Could you check a few things on this model? Use its own coordinates, in mm. Give positions to 0.01 mm unless a question says otherwise; leave off trailing zeros. Write each loop counter-clockwise with the first axis right and the second up, starting at its lowest first coordinate (ties: lowest second). Pieces come first, ordered by that corner, then holes. Notation, with made-up numbers: (51.5, -21.5) - (80.5, -21.5) arc R10 cw to (80.5, -7.5) - close; hole circle Ø6 at (-15.75, -17). An arc over 180 degrees is marked (long way). Answer as CSV lines item,"result". Start each with the question number.
Q1. Imagine slicing it at A-A on x = 18. List the corners of the cut face in (y, z) for me (3 decimals).
Q2. Imagine slicing it at D-D on z = 1. State how many separate pieces and enclosed holes the cut face has, and give its area (3 significant figures).
Q3. We'd pull the mould along Y, two halves only. Please class faces 1 (the face through (-35, 27, 0)), 2 (the face through (-92.41, 108.18, 1)): pulls with the +Y half, pulls with the -Y half, needs draft (parallel to the pull), parting line crosses it, or undercut.
Q4. Imagine slicing it at B-B on x = 70.5. List the corners of the cut face in (y, z) for me (3 decimals), and give its area (3 significant figures).
Q5. Imagine slicing it at C-C on y = 37.5. List the corners of the cut face in (x, z) for me.
Q6. If I drill on line 1 along Y through (x, z) = (7, 0.6) (3 decimals); line 2 along Y through (x, z) = (-69, 0.4) (3 decimals); line 3 along X through (y, z) = (12, 1.5), over which ranges is the centre line in solid material (lowest first)?
```python
from build123d import *

# Parameters (mm, degrees)
F0_R     = 1.524
F0_W     = 222.25
F0_H     = 11.1252
F0_R_2   = 2.5654
F0_R_3   = 4.3815
F0_W_2   = 44.5262
F0_H_2   = 60.96
F1_DEPTH = 2.032
F2_R     = 5.08


with BuildPart() as f1:
    # F0 (on Top) → F1 (new body)
    with BuildSketch(Plane.XY):
        Polygon((-146.177, 82.296), (-146.177, -82.296), (146.177, -82.296), (146.177, 82.296), (121.285, 82.296), (121.285, 133.096), (-121.285, 133.096), (-121.285, 82.296), align=None)
        with Locations((-107.188, -65.6336)):
            Circle(F0_R, mode=Mode.SUBTRACT)
        with Locations((-107.188, -35.6616)):
            Circle(F0_R, mode=Mode.SUBTRACT)
        with Locations((-3.556, -50.9524)):
            Rectangle(F0_W, F0_H, mode=Mode.SUBTRACT)
        with Locations((-30.4038, -2.7686)):
            Circle(F0_R_2, mode=Mode.SUBTRACT)
        with Locations((107.569, -65.6336)):
            Circle(F0_R, mode=Mode.SUBTRACT)
        with Locations((107.569, -35.5854)):
            Circle(F0_R, mode=Mode.SUBTRACT)
        with Locations((30.4038, -2.7686)):
            Circle(F0_R_2, mode=Mode.SUBTRACT)
        with Locations((-28.998554, 60.7314)):
            Circle(F0_R_2, mode=Mode.SUBTRACT)
        with Locations((-88.03132, 107.9881)):
            Circle(F0_R_3, mode=Mode.SUBTRACT)
        with Locations((0.2159, 25.5524)):
            Rectangle(F0_W_2, F0_H_2, mode=Mode.SUBTRACT)
        with Locations((28.998554, 60.7314)):
            Circle(F0_R_2, mode=Mode.SUBTRACT)
        with Locations((88.03132, 107.9881)):
            Circle(F0_R_3, mode=Mode.SUBTRACT)
    extrude(amount=F1_DEPTH)

    # F2
    f2_edges = [f1.edges().sort_by_distance(p)[0] for p in [
        (121.285, 133.096, 1.016),
        (-121.285, 133.096, 1.016),
        (146.177, -82.296, 1.016),
        (-146.177, -82.296, 1.016),
    ]]
    fillet(f2_edges, radius=F2_R)


solid = f1.part
```
Conclusion:
1,outline,"(-82.296, 0) - (-56.515, 0) - (-56.515, 2.032) - (-82.296, 2.032) - close; (-45.39, 0) - (-4.928, 0) - (-4.928, 2.032) - (-45.39, 2.032) - close; (56.032, 0) - (133.096, 0) - (133.096, 2.032) - (56.032, 2.032) - close"
2,separate pieces,"1"
2,enclosed holes,"12"
2,area,"55,000 mm^2"
3,face 1,"needs draft"
3,face 2,"undercut"
4,outline,"(-82.296, 0) - (-56.515, 0) - (-56.515, 2.032) - (-82.296, 2.032) - close; (-45.39, 0) - (133.096, 0) - (133.096, 2.032) - (-45.39, 2.032) - close"
4,area,"415 mm^2"
5,outline,"(-146.18, 0) - (-22.05, 0) - (-22.05, 2.03) - (-146.18, 2.03) - close; (22.48, 0) - (146.18, 0) - (146.18, 2.03) - (22.48, 2.03) - close"
6,line 1,"-82.296 to -56.515, -45.39 to -4.928, 56.032 to 133.096"
6,line 2,"-82.296 to -56.515, -45.39 to 133.096"
6,line 3,"-146.18 to -22.05, 22.48 to 146.18"
